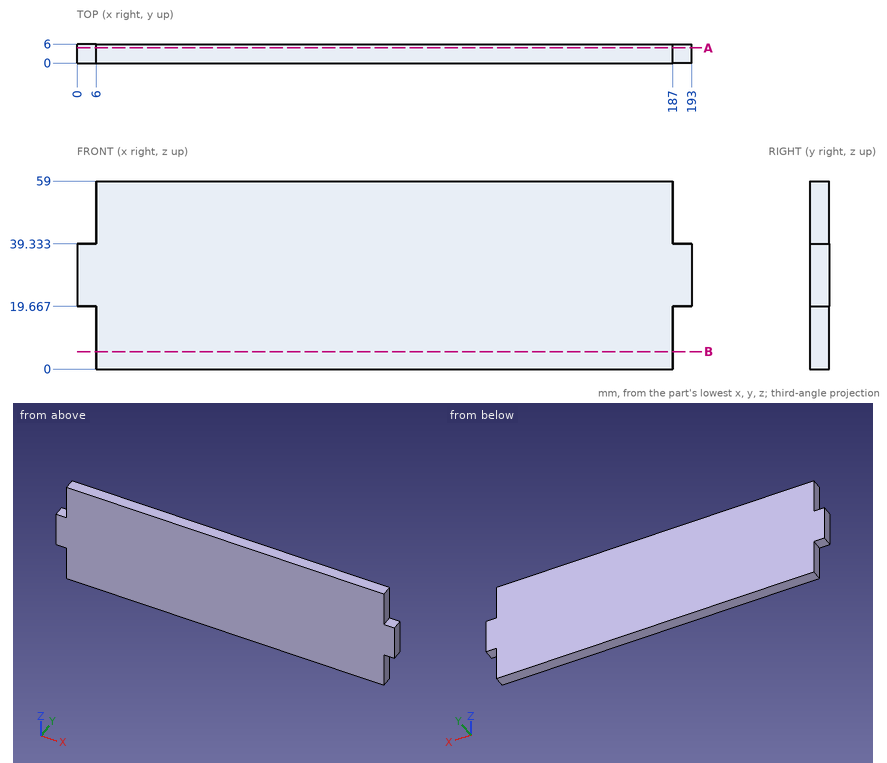
The figure shows three views and two pictorial views of one solid part (mm, origin at its lowest corner). Answer the questions. Coordinates: 2 decimals unless noted, no trailing zeros. Loops run counter-clockwise (first coordinate to the right, second up) from the corner with the lowest first, then second, coordinate; pieces in that order, holes last. Notation, with made-up numbers: (73, 84) -> (99, 84) arc R28 cw to (99, 103) -> close; hole circle Ø9 at (83.5, 40). An arc over 180 degrees is marked (long way). Return JSON: item names as keys, results as strings. Group by question number.
(1) Find the intervals of material crossed by probe 1 along X at (y, z) = (4.4, 17.5), in increasing order. Write a range as from..to.
(2) A cutting plane is placed at A-A on y = 4.8. Write down the section's boundary in (x, z).
(3) A cutting plane is placed at B-B on z = 5.5. Write down the section's boundary in (x, y).
(4) Given pin 1 Ø12 at (x, z) = (32.5, 17.5) entering from -Y; pin 2 Ø1.8 at (y, z) = (3, 8) entering from -X; pin 3 Ø1.8 at (y, z) = (3.5, 48.5) entering from +X; pin 4 Ø1.8 at (x, y) = (2.5, 3.5) entering from -Z, each flat-ended and moving along its own axis, determine where each tip first touches the part or whether it passes through.
The answers:
{
 "1": {"probe 1": "x = 6..187"},
 "2": {"outline": "(0, 19.67) -> (6, 19.67) -> (6, 0) -> (187, 0) -> (187, 19.67) -> (193, 19.67) -> (193, 39.33) -> (187, 39.33) -> (187, 59) -> (6, 59) -> (6, 39.33) -> (0, 39.33) -> close"},
 "3": {"outline": "(6, 0) -> (187, 0) -> (187, 6) -> (6, 6) -> close"},
 "4": {"pin 1": "stops at y = 0", "pin 2": "stops at x = 6", "pin 3": "stops at x = 187", "pin 4": "stops at z = 19.67"}
}
